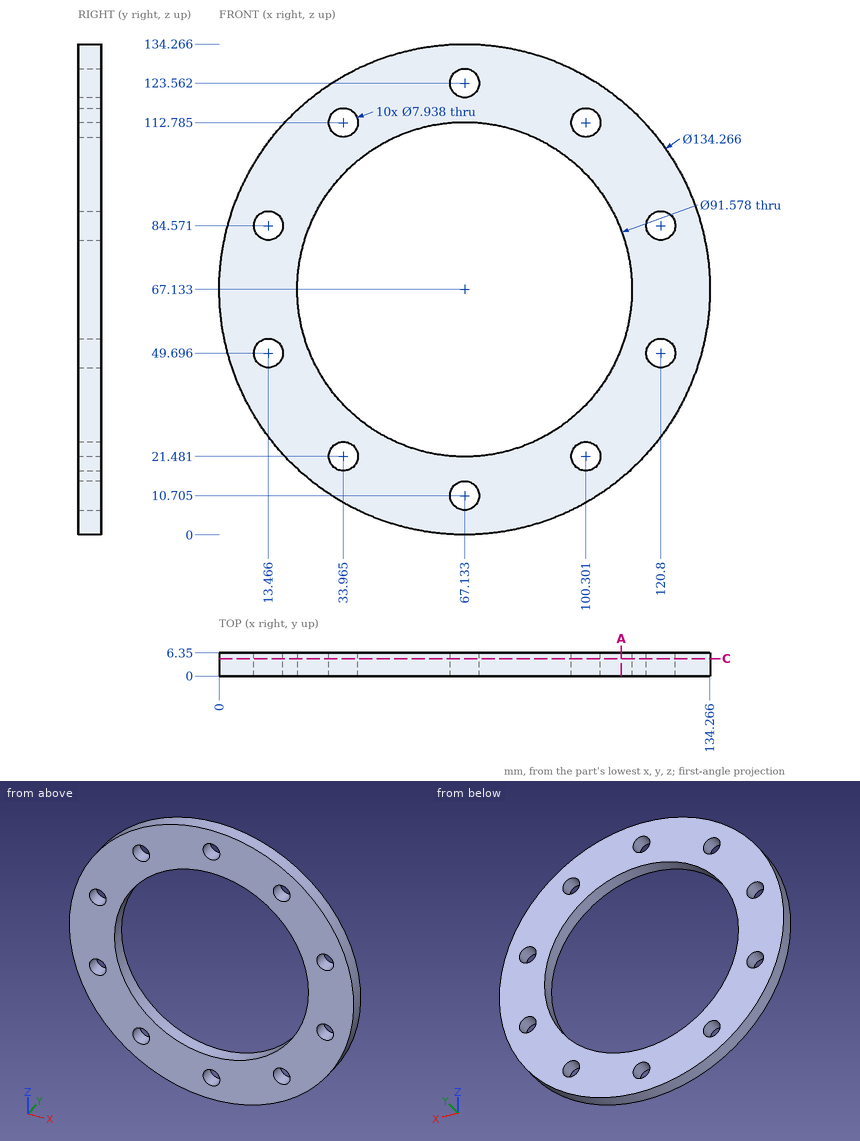
The figure shows three views and two pictorial views of one solid part (mm, origin at its lowest corner). Answer the questions. Give positions to 0.01 mm unless a question says otherwise; leave off trailing zeros. Write each loop counter-clockwise with the first axis right and the second up, starting at its lowest first coordinate (ties: lowest second). Pieces come first, ordered by that corner, then holes. Notation, with made-up numbers: M 42,-38 L 101,-38 A32 ccw 101,-1 Z; hole C 40.5,41.5 d7. An arc over 180 degrees is marked long. One line per item, written item: value. Start each with the question number.
(1) Find section C-C (y = 4.75). Give the number of separate pieces and of enclosed holes in the cut face, plus the area to 3 significant figures.
(2) Find section A-A (x = 110). Determine the outline of the cut face in (y, z).
(3) Find the intervals of material crossed by line 1 (X direction, y = 2.5, z = 85) (1 decimal); line 2 (X direction, y = 2.5, z = 114.5) (1 decimal); line 3 (Z direction, x = 83, y = 5.75) (1 decimal), in increasing order.
(4) Flat-ended cylindrical pins translate along their axes: pin 1 Ø7 at (x, z) = (33.97, 112.78) entering from -Y; pin 2 Ø3 at (y, z) = (4, 49) entering from -X; pin 3 Ø1.5 at (x, y) = (80, 2) entering from +Z. Find the tip coordinate at first contact, or state that the pin passes through.
Results below:
1. separate pieces: 1
1. enclosed holes: 11
1. area: 7,080 mm^2
2. outline: M 0,15.47 L 6.35,15.47 L 6.35,51.04 L 0,51.04 Z; M 0,83.23 L 6.35,83.23 L 6.35,118.8 L 0,118.8 Z
3. line 1: x = 2.4 to 9.5, 17.4 to 25, 109.3 to 116.9, 124.7 to 131.8
3. line 2: x = 19.6 to 30.4, 37.5 to 96.7, 103.9 to 114.7
3. line 3: z = 1.9 to 24.2, 110.1 to 132.4
4. pin 1: passes through
4. pin 2: stops at x = 2.09
4. pin 3: stops at z = 133.16
